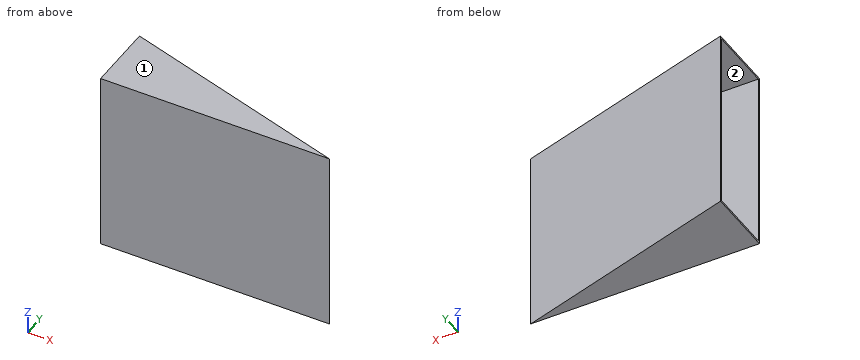
from build123d import *

# Parameters (mm, degrees)
BOSS_EXTRUDE1_DEPTH = 609.6
SHELL1_T            = -6.35


with BuildPart() as part:
    # Sketch1 → Boss-Extrude1 (new body)
    with BuildSketch(Plane.XY):
        Polygon((0, 228.6), (0, 0), (762, 0), align=None)
    extrude(amount=-BOSS_EXTRUDE1_DEPTH)

    # Shell1
    shell1_openings = [part.faces().sort_by_distance(p)[0] for p in [
        (0, 114.3, -304.8),
    ]]
    offset(amount=SHELL1_T, openings=shell1_openings, kind=Kind.INTERSECTION)


solid = part.part
Check sheet for the modelled part. Datum: model origin and axes. Units: mm. Face numbers are marked on the shaded views. A direction names the side the tool comes from. Round coordinates to 2 decimals unless told otherwise and drop trailing zeros. Loops run counter-clockwise (first coordinate to the right, second up) from the corner with the lowest first, then second, coordinate; pieces in that order, holes last. Notation, with made-up numbers: M 1.25,68 L 17.25,68 A27 ccw 17.25,95 Z; hole C 88.25,-12.5 d10. An arc over 180 degrees is marked long. One line per item, written item: value.
(1) Depth check by flat-ended pin: pin 1 Ø4 at (x, z) = (444.5, -454.5) entering from -Y; pin 2 Ø1 at (x, z) = (439.5, -333) entering from +Y. Enter the tip coordinate at first touch or a pass-through.
Computed values:
pin 1: stops at y = 0
pin 2: stops at y = 96.9
(2) Access from +Z, -Z, +X, -X, +Y, -Y to the whole of each face (thin tool, end or side, straight path). Record for the marked faces 1 and 2.
Computed values:
face 1: +Z, +X, -X, +Y, -Y
face 2: -X
(3) Thickness scan on line 1 (Z direction, x = 407, y = 70); line 2 (Y direction, x = 89, z = -562). Record the ranges inside material, lowest first.
Computed values:
line 1: z = -609.6 to -603.25, -6.35 to 0
line 2: y = 0 to 6.35, 195.27 to 201.9
(4) Sectioned sample at B-B, the plane z = -112.5. Record the cut outline in (x, y).
Computed values:
outline: M 0,0 L 762,0 L 0,228.6 L 0,221.97 L 718.73,6.35 L 0,6.35 Z
(5) Sectioned sample at D-D, the plane x = 426.5. Record the cut outline in (y, z), then the cut area to 3 significant figures.
Computed values:
outline: M 0,-609.6 L 100.65,-609.6 L 100.65,0 L 0,0 Z; hole M 6.35,-603.25 L 94.02,-603.25 L 94.02,-6.35 L 6.35,-6.35 Z
area: 9,030 mm^2
(6) Sectioned sample at A-A, the plane x = 542.5. Record the cut outline in (y, z).
Computed values:
outline: M 0,-609.6 L 65.85,-609.6 L 65.85,0 L 0,0 Z; hole M 6.35,-603.25 L 59.22,-603.25 L 59.22,-6.35 L 6.35,-6.35 Z
(7) Sectioned sample at C-C, the plane y = 192. Record the cut outline in (x, z).
Computed values:
outline: M 0,-609.6 L 122,-609.6 L 122,0 L 0,0 L 0,-6.35 L 99.9,-6.35 L 99.9,-603.25 L 0,-603.25 Z
